Autodesk Inventor part; units mm, degrees
ref_plane "YZ Plane" through (0, 0, 0) normal (1, 0, 0) x (0, 1, 0)
ref_plane "XZ Plane" through (0, 0, 0) normal (0, 1, 0) x (-1, 0, 0)
ref_plane "XY Plane" through (0, 0, 0) normal (0, 0, 1) x (1, 0, 0)
sketch "Sketch1" plane through (0, 0, 0) normal (0, 1, 0) x (-1, 0, 0)
  line L0 (-90.75, 80) -> (90.75, 80)
  line L1 (90.75, 80) -> (90.75, -80)
  line L2 (90.75, -80) -> (-90.75, -80)
  line L3 (-90.75, -80) -> (-90.75, 80)
  line L4 (-90.75, 80) -> (90.75, -80) construction
  line L5 (90.75, 80) -> (-90.75, -80) construction
  point P0 (0, 0)
  dimension "d0" = 181.5
  dimension "d1" = 160
extrude "Extrusion1" add sketch "Sketch1" along normal blind 1
sketch "Sketch2" plane through (-89.75, 0, 80) normal (-1, 0, 0) x (0, -1, 0)
  line L0 (0, -160) -> (0, 0)
  line L1 (0, 0) -> (-117.5, 0)
  line L2 (-117.5, 0) -> (-117.5, -160)
  line L3 (-117.5, -160) -> (0, -160)
edge flange "Flange1" height 117.5 angle 90 thickness 1 bend radius 1 thickness toward (-1, 0, 0) relief tear relief width 1 relief depth 0.5 edges at (-90.75, 1, 0) wall of the first edge with corners at (-89.75, 0, -80) (-89.75, 0, 80) (-89.75, 117.5, 80) (-89.75, 117.5, -80)
bend "Bend1"
corner "Corner1"
sketch "Sketch3" plane through (-90.25, 116.634, 80) normal (0.5, 0.8660254, 0) x (0.8660254, -0.5, 0)
  line L0 (0, -160) -> (0, 0)
  line L1 (0, 0) -> (-10, 0)
  line L2 (-10, 0) -> (-10, -160)
  line L3 (-10, -160) -> (0, -160)
edge flange "Flange2" height 10 angle -60 thickness 1 bend radius 1 thickness toward (0.5, 0.8660254, 0) relief tear relief width 1 relief depth 0.5 edges at (-89.75, 117.5, 0) wall of the first edge with corners at (-90.25, 116.634, -80) (-90.25, 116.634, 80) (-98.9103, 121.634, 80) (-98.9103, 121.634, -80)
bend "Bend2"
corner "Corner2"
sketch "Sketch4" plane through (-98.4103, 122.5, 80) normal (0.5, 0.8660254, 0) x (0, 0, -1)
  line L0 (160, 0) -> (0, 0)
  line L1 (80, 0) -> (80, -5)
  line L2 (80, 0) -> (85, 0) construction
  line L3 (80, -5) -> (155, -5)
  line L4 (80, -5) -> (155, -5) construction
  line L5 (80, -5) -> (5, -5)
  line L6 (80, -5) -> (155, -5) construction
  point P0 (80, -146.4758)
  dimension "d25" = 5
  dimension "d26" = 90
  dimension "d27" = 75
  dimension "d28" = 0
  dimension "d29" = 75
  dimension "d30" = 180
hole "Hole1" at (-94.0801, 120, 75) at (-94.0801, 120, -75) direction (-0.5, -0.8660254, 0) diameter 4.5 depth 1 tip angle 118
sketch "Sketch5" plane through (89.884, 0.5, -80) normal (0.8660254, -0.5, 0) x (0.5, 0.8660254, 0)
  line L0 (0, 160) -> (0, 0)
  line L1 (0, 0) -> (31.5, 0)
  line L2 (31.5, 0) -> (31.5, 160)
  line L3 (31.5, 160) -> (0, 160)
edge flange "Flange3" height 31.5 angle 60 thickness 1 bend radius 1 thickness toward (0.8660254, -0.5, 0) relief tear relief width 1 relief depth 0.5 edges at (90.75, 1, 0) wall of the first edge with corners at (89.884, 0.5, 80) (89.884, 0.5, -80) (105.634, 27.7798, -80) (105.634, 27.7798, 80)
bend "Bend3"
corner "Corner3"
sketch "Sketch6" plane through (106.5, 27.2798, 80) normal (0.8660254, -0.5, 0) x (0, 0, -1)
  line L0 (0, 0) -> (160, 0)
  line L1 (80, 0) -> (80, -10)
  line L2 (80, 0) -> (90, 0) construction
  point P0 (80, -76.875)
  dimension "d48" = 10
  dimension "d49" = 90
hole "Hole3" at (101.5, 18.6195, 0) direction (-0.8660254, 0.5, 0) diameter 4.5 depth 1 tip angle 118
sketch "Sketch7" plane through (0, 0, 0) normal (0, -1, 0) x (1, 0, 0)
  line L0 (89.5953, -80) -> (89.5953, 80)
  line L1 (-88.75, 80) -> (89.5953, 80)
  line L2 (-88.75, 80) -> (-88.75, -80)
  line L3 (89.5953, -80) -> (-88.75, -80)
  line L4 (-88.75, 80) -> (-68.75, 80)
  line L5 (-88.75, 80) -> (89.5953, 80)
  line L6 (-68.75, 80) -> (-68.75, 60)
  line L7 (-88.75, 0) -> (89.5953, 0)
  line L8 (0.4226, 80) -> (0.4226, -80)
  point P0 (0, 0)
  point P1 (-68.75, -60)
  point P2 (69.5953, 60)
  point P3 (69.5953, -60)
  dimension "d67" = 20
  dimension "d68" = 20
hole "Hole4" at (69.5953, 0, -60) at (-68.75, 0, -60) at (-68.75, 0, 60) at (69.5953, 0, 60) direction (0, 1, 0) diameter 5 depth 1 tip angle 118
equation "\"d36\" = Thickness"
equation "\"d65\" = Thickness"
equation "\"d74\" = Thickness"
equation "\"d4\" = Thickness"
equation "\"d5\" = BendReliefWidth"
equation "\"d6\" = BendReliefDepth"
equation "\"d7\" = MinimumRemnant"
equation "\"d8\" = TransitionRadius"
equation "\"d11\" = BendRadius"
equation "\"d12\" = CornerReliefSize"
equation "\"d13\" = GapSize"
equation "\"d14\" = JacobiRadiusSize"
equation "\"d15\" = BendReliefWidth"
equation "\"d16\" = BendReliefDepth"
equation "\"d17\" = MinimumRemnant"
equation "\"d18\" = TransitionRadius"
equation "\"d21\" = BendRadius"
equation "\"d22\" = CornerReliefSize"
equation "\"d23\" = GapSize"
equation "\"d24\" = JacobiRadiusSize"
equation "\"d38\" = BendReliefWidth"
equation "\"d39\" = BendReliefDepth"
equation "\"d40\" = MinimumRemnant"
equation "\"d41\" = TransitionRadius"
equation "\"d44\" = BendRadius"
equation "\"d45\" = CornerReliefSize"
equation "\"d46\" = GapSize"
equation "\"d47\" = JacobiRadiusSize"
equation "\"BendRadius\" = Thickness"
equation "\"BendReliefWidth\" = Thickness"
equation "\"BendReliefDepth\" = 0.5 * Thickness"
equation "\"CornerReliefSize\" = 4 * Thickness"
equation "\"MinimumRemnant\" = 2 * Thickness"
equation "\"TransitionRadius\" = BendRadius"
equation "\"JacobiRadiusSize\" = BendRadius"
equation "\"GapSize\" = Thickness"
properties part number "zetdeel_hoog" material "Steel, Galvanized"
Input: part model. Units: mm. Frame: model coordinates. A direction names the side the tool comes from. Coordinates: 2 decimals unless noted, no trailing zeros. Loops run counter-clockwise (first coordinate to the right, second up) from the corner with the lowest first, then second, coordinate; pieces in that order, holes last. Notation, with made-up numbers: (13.5, 30.5) -> (66.5, 30.5) arc R33 cw to (66.5, 64.5) -> close; hole circle Ø6 at (33, 55.25). An arc over 180 degrees is marked (long way). Write item = value, one per line. Start each with the question number.
Item 1: Cut plane A-A, the plane z = -60. Return loops of the section in (x, y), plus the area to 3 significant figures.
Item 2: Mould query, pull axis X, two halves, no side actions, for faces 3 (the face through (-67.79, 0.51, -62.31)), 4 (the face through (-94.6, 120.3, -1.1)), 5 (the face through (-90.75, 60, 1)), 6 (the face through (2, 0, 1)). Classes: pulls with the +X half, pulls with the -X half, needs draft (parallel to the pull), parting line crosses it, or undercut.
Item 3: Reachability of faces 1 (the face through (-94.919, 119.899, -72.854)), 2 (the face through (97.941, 14.456, -1.12)) from +Z, -Z, +X, -X, +Y, -Y: full face, straight path, thin tool, end or side. Return the list, or none.
Item 4: Cut plane C-C, the plane y = 10. Return loops of the section in (x, z), plus the area to 3 significant figures.
Item 5: Material intervals for line 1 (Z direction, x = -68.75, y = 0.5); line 2 (Y direction, x = 31, z = 52.5); line 3 (X direction, y = 96.5, z = -38), sorted ascending.
Item 6: Cut plane D-D, the plane z = 54. Return loops of the section in (x, y).
Item 7: First-contact query: P1, Ø12, axis at y = 57.5, z = 18, coming from the +X side; P2, Ø6, axis at x = 9.5, z = -43.5, coming from the +Y side; P3, Ø8, axis at y = 68.5, z = -61, coming from the -X side. Flat tips, straight axial feed; report the tip coordinate or a pass-through.
Item 8: Cut plane B-B, the plane x = -68.75. Return loops of the section in (y, z), plus the area to 3 significant figures.
Ans:
q1.outline = (-98.91, 121.63) -> (-91.25, 117.21) arc R1 cw to (-90.75, 116.35) -> (-90.75, 2) arc R2 ccw to (-88.75, 0) -> (-71.25, 0) -> (-71.25, 1) -> (-88.75, 1) arc R1 cw to (-89.75, 2) -> (-89.75, 116.35) arc R2 ccw to (-90.75, 118.08) -> (-98.41, 122.5) -> close; (-66.25, 0) -> (67.1, 0) -> (67.1, 1) -> (-66.25, 1) -> close; (72.1, 0) -> (89.6, 0) arc R2 ccw to (91.33, 1) -> (106.5, 27.28) -> (105.63, 27.78) -> (90.46, 1.5) arc R1 cw to (89.6, 1) -> (72.1, 1) -> close
q1.area = 327 mm²
q2.face_3 = undercut
q2.face_4 = pulls with the +X half
q2.face_5 = pulls with the -X half
q2.face_6 = needs draft
q3.face_1 = none
q3.face_2 = +Z, -Z, +Y
q4.outline = (-90.75, -80) -> (-89.75, -80) -> (-89.75, 80) -> (-90.75, 80) -> close; (95.37, -80) -> (96.52, -80) -> (96.52, 80) -> (95.37, 80) -> close
q4.area = 345 mm²
q5.line_1 = -80 to -62.5, -57.5 to 57.5, 62.5 to 80
q5.line_2 = 0 to 1
q5.line_3 = -90.75 to -89.75
q6.outline = (-98.91, 121.63) -> (-91.25, 117.21) arc R1 cw to (-90.75, 116.35) -> (-90.75, 2) arc R2 ccw to (-88.75, 0) -> (89.6, 0) arc R2 ccw to (91.33, 1) -> (106.5, 27.28) -> (105.63, 27.78) -> (90.46, 1.5) arc R1 cw to (89.6, 1) -> (-88.75, 1) arc R1 cw to (-89.75, 2) -> (-89.75, 116.35) arc R2 ccw to (-90.75, 118.08) -> (-98.41, 122.5) -> close
q7.P1 = -89.75
q7.P2 = 1
q7.P3 = -90.75
q8.outline = (0, -80) -> (1, -80) -> (1, -62.5) -> (0, -62.5) -> close; (0, -57.5) -> (1, -57.5) -> (1, 57.5) -> (0, 57.5) -> close; (0, 62.5) -> (1, 62.5) -> (1, 80) -> (0, 80) -> close
q8.area = 150 mm²
